The model under review builds one solid part; all positions refer to its coordinate system, in mm. A direction names the side the tool comes from. Round coordinates to 2 decimals unless told otherwise and drop trailing zeros. Write each loop counter-clockwise with the first axis right and the second up, starting at its lowest first coordinate (ties: lowest second). Pieces come first, ordered by that corner, then holes. Notation, with made-up numbers: (49.5, 22) - (81.5, 22) arc R21 ccw to (81.5, 37) - close; hole circle Ø11 at (-20, 76.25). An arc over 180 degrees is marked (long way). Use one line per item in the form item = value.
from build123d import *

# Parameters (mm, degrees)
SKETCH1_R               = 1.5
SKETCH1_R_2             = 7.95
MAIN_BODY_LINK_B1_DEPTH = 3
CUT_EXTRUDE1_REACH      = 168.945
CUT_EXTRUDE2_REACH      = 168.945
SKETCH3_R               = 1.5
FILLET1_R               = 1


with BuildPart() as part:
    # Sketch1 → Main Body Link B1 (new body)
    with BuildSketch(Plane.XY):
        with BuildLine():
            Line((-11.1, 83.474052381), (-9.1, 83.474052381))
            Line((-9.1, 83.474052381), (0, 83.474052381))
            Line((0, 83.474052381), (9.1, 83.474052381))
            Line((9.1, 83.474052381), (11.1, 83.474052381))
            Line((11.1, 83.474052381), (20.2, 83.474052381))
            Line((20.2, 83.474052381), (20.2, 90.874052381))
            Line((20.2, 90.874052381), (17.986683974, 148.383116621))
            ThreePointArc((17.986683974, 148.383116621), (0, 165.690874165), (-17.986683974, 148.383116621))
            Line((-17.986683974, 148.383116621), (-20.2, 90.874052381))
            Line((-20.2, 90.874052381), (-20.2, 83.474052381))
            Line((-20.2, 83.474052381), (-11.1, 83.474052381))
        make_face()
        with Locations((5.2, 88.124052381)):
            Circle(SKETCH1_R, mode=Mode.SUBTRACT)
        with Locations((15, 88.124052381)):
            Circle(SKETCH1_R, mode=Mode.SUBTRACT)
        with Locations((-15, 88.124052381)):
            Circle(SKETCH1_R, mode=Mode.SUBTRACT)
        with Locations((-5.2, 88.124052381)):
            Circle(SKETCH1_R, mode=Mode.SUBTRACT)
        with Locations((0, 147.690874165)):
            Circle(SKETCH1_R_2, mode=Mode.SUBTRACT)
    extrude(amount=MAIN_BODY_LINK_B1_DEPTH)

    # Sketch2 → Cut-Extrude1 (cut, up to next)
    with BuildSketch(Plane.XY.offset(3), mode=Mode.PRIVATE) as cut_extrude1_sk1:
        Polygon((-3.278172542, 117.482670232), (12, 128.172168466), (12, 106.793171999), align=None)
    cut_extrude1_tool1 = extrude(cut_extrude1_sk1.sketch, amount=-CUT_EXTRUDE1_REACH, mode=Mode.PRIVATE) & part.part
    # Sketch2 → Cut-Extrude1 (cut, up to next)
    with BuildSketch(Plane.XY.offset(3), mode=Mode.PRIVATE) as cut_extrude1_sk2:
        with BuildLine():
            ThreePointArc((-12, 134.2744663), (-7.774454217, 131.456408925), (-2.929911079, 129.930929878))
            Line((-2.929911079, 129.930929878), (-12, 123.584968066))
            Line((-12, 123.584968066), (-12, 134.2744663))
        make_face()
    cut_extrude1_tool2 = extrude(cut_extrude1_sk2.sketch, amount=-CUT_EXTRUDE1_REACH, mode=Mode.PRIVATE) & part.part
    # Sketch2 → Cut-Extrude1 (cut, up to next)
    with BuildSketch(Plane.XY.offset(3), mode=Mode.PRIVATE) as cut_extrude1_sk3:
        Polygon((-12, 111.380372399), (-12, 100.690874165), (3.278172542, 100.690874165), align=None)
    cut_extrude1_tool3 = extrude(cut_extrude1_sk3.sketch, amount=-CUT_EXTRUDE1_REACH, mode=Mode.PRIVATE) & part.part
    add(cut_extrude1_tool1.solids().sort_by_distance((6.907276, 117.48267, 3))[0], mode=Mode.SUBTRACT)
    add(cut_extrude1_tool2.solids().sort_by_distance((-9.12997, 128.978342, 3))[0], mode=Mode.SUBTRACT)
    add(cut_extrude1_tool3.solids().sort_by_distance((-6.907276, 104.25404, 3))[0], mode=Mode.SUBTRACT)

    # Sketch3 → Cut-Extrude2 (cut, up to next)
    with BuildSketch(Plane.XY.offset(3), mode=Mode.PRIVATE) as cut_extrude2_sk1:
        with Locations((-11.5, 147.690874165)):
            Circle(SKETCH3_R)
    cut_extrude2_tool1 = extrude(cut_extrude2_sk1.sketch, amount=-CUT_EXTRUDE2_REACH, mode=Mode.PRIVATE) & part.part
    # Sketch3 → Cut-Extrude2 (cut, up to next)
    with BuildSketch(Plane.XY.offset(3), mode=Mode.PRIVATE) as cut_extrude2_sk2:
        with Locations((11.5, 147.690874165)):
            Circle(SKETCH3_R)
    cut_extrude2_tool2 = extrude(cut_extrude2_sk2.sketch, amount=-CUT_EXTRUDE2_REACH, mode=Mode.PRIVATE) & part.part
    add(cut_extrude2_tool1.solids().sort_by_distance((-11.5, 147.690874, 3))[0], mode=Mode.SUBTRACT)
    add(cut_extrude2_tool2.solids().sort_by_distance((11.5, 147.690874, 3))[0], mode=Mode.SUBTRACT)

    # Fillet1
    fillet1_edges = [part.edges().sort_by_distance(p)[0] for p in [
        (-3.278172542, 117.482670232, 1.5),
        (12, 128.172168466, 1.5),
        (12, 106.793171999, 1.5),
        (-12, 134.2744663, 1.5),
        (-2.929911079, 129.930929878, 1.5),
        (-12, 123.584968066, 1.5),
        (-12, 111.380372399, 1.5),
        (3.278172542, 100.690874165, 1.5),
        (-12, 100.690874165, 1.5),
    ]]
    fillet(fillet1_edges, radius=FILLET1_R)


solid = part.part
(1) Add section C-C on z = 1.05. Count the separate pieces of the cut face and the enclosed holes in it, then the cut area to 3 significant figures.
Geometry results:
separate_pieces = 1
enclosed_holes = 10
area = 2,460 mm2
(2) The part is to be moulded in two halves that separate along Y. For faces 1 (the flat face through (-19.078, 120.031, 1.479)), 2 (the flat face through (12, 118, 2)), 3 (the flat face through (0, 125, 3)), say which applies: +Y half, -Y half, draft (parallel to the pull), parting line (faces both ways), or undercut.
Geometry results:
face_1 = +Y half
face_2 = undercut
face_3 = draft
(3) Add section B-B on x = 15. Write out the cut boundary in (y, z).
Geometry results:
outline = (83.47, 0) - (86.62, 0) - (86.62, 3) - (83.47, 3) - close; (89.62, 0) - (157.64, 0) - (157.64, 3) - (89.62, 3) - close
(4) Add section A-A on y = 152. Write out the cut boundary in (x, z).
Geometry results:
outline = (-17.48, 0) - (-6.68, 0) - (-6.68, 3) - (-17.48, 3) - close; (6.68, 0) - (17.48, 0) - (17.48, 3) - (6.68, 3) - close
(5) To check wall thickness, follow L1, parallel to Y at x = 3.5, z = 0.35; L2, parallel to Y at x = -11, z = 1.45; L3, parallel to Y at x = 4.5, z = 2.3. State the ranges of each line that lie inside material, in increasing order.
Geometry results:
L1 = 83.47 to 112.74, 122.23 to 140.55, 154.83 to 165.35
L2 = 83.47 to 100.69, 110.46 to 124.51, 133.2 to 146.28, 149.11 to 161.94
L3 = 83.47 to 86.8, 89.45 to 112.04, 122.92 to 141.14, 154.24 to 165.12
(6) Machinability: for faces 4 (the flat face through (-20.2, 87, 1)), 5 (the cylindrical face through (1.05, 101.37, 1.48)), which of the approach directions +Z, -Z, +X, -X, +Y, -Y give a long, thin tool a straight path to every point of the face, cutting with its end or side? Answer none if there is none.
Geometry results:
face_4 = +Z, -Z, -X, +Y, -Y
face_5 = +Z, -Z
(7) Insertion check: P1, Ø1.5, axis at y = 105, z = 2, coming from the +X side; P2, Ø0.9, axis at x = -4, z = 1, coming from the +Y side; P3, Ø0.9, axis at y = 127.5, z = 1, coming from the +X side. Each pin has a flat end and moves straight along its axis. Give the tip position at first contact, or say it passes through.
Geometry results:
P1 = 19.69
P2 = 165.34
P3 = 18.81
(8) Add section D-D on y = 138. Write out the cut boundary in (x, z), then the cut area to 3 significant figures.
Geometry results:
outline = (-18.39, 0) - (18.39, 0) - (18.39, 3) - (-18.39, 3) - close
area = 110 mm2
